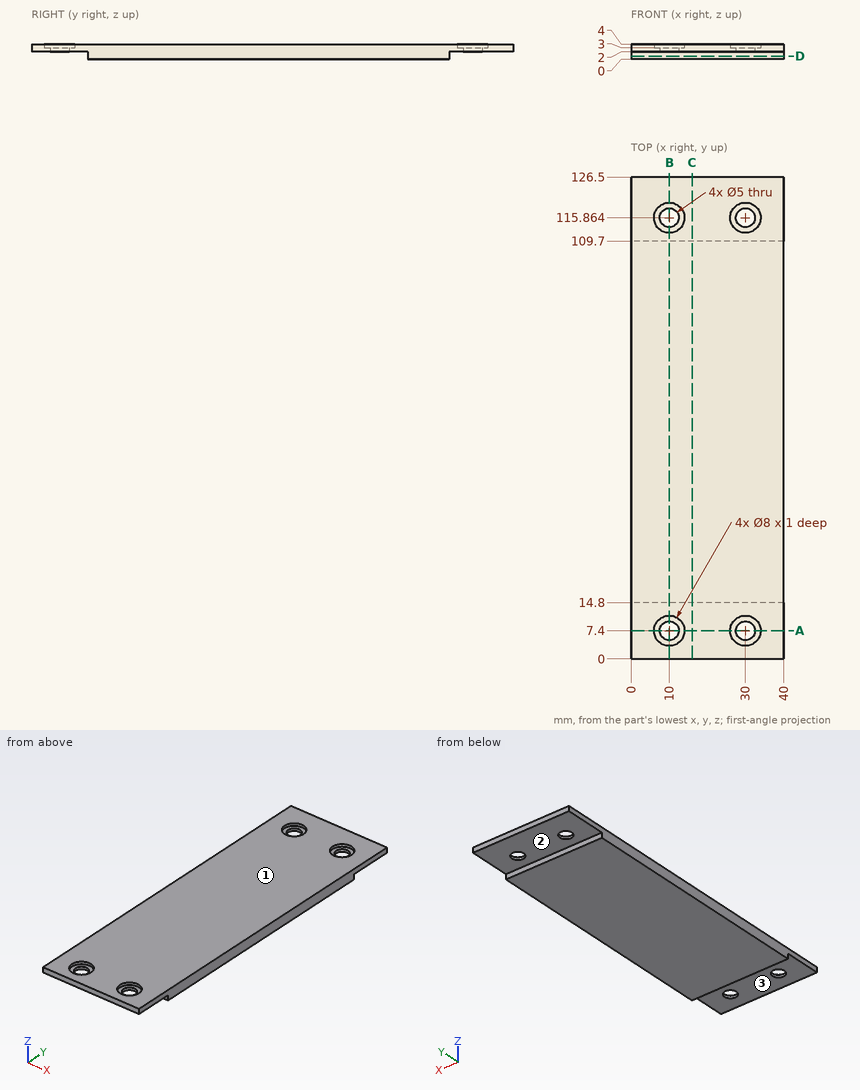
Could you check a few things on this drawing? It's one solid part, dimensions in mm from its lowest x, y, z. A direction names the side the tool comes from. Give positions to 0.01 mm unless a question says otherwise; leave off trailing zeros. Order: outer loops, then holes, each group sorted by start corner. A loop starts at its lowest first (then second) coordinate and runs counter-clockwise, first axis right, second up. Notation, with made-up numbers: (14, 67) - (27, 67) arc R24 cw to (27, 96) - close; hole circle Ø2 at (-1, -10.75). An arc over 180 degrees is marked (long way). One line per question, with ' | ' between items. Start each with the question number.
Item 1: For the marked faces 1, 2 and 3, which set-ups out of +Z, -Z, +X, -X, +Y, -Y let a thin tool reach every point of the face, with its end or its side?
Item 2: I want a section at D-D on z = 0.8. Write out the boundary of the cut face in (x, y), then the cut area to 3 significant figures.
Item 3: I want a section at C-C on x = 16. Write out the boundary of the cut face in (y, z).
Item 4: I want a section at A-A on y = 7.4. Write out the boundary of the cut face in (x, z), then the cut area to 3 significant figures.
Item 5: I want a section at B-B on x = 10. Write out the boundary of the cut face in (y, z).
Item 6: I need wall thicknesses on probe 1 along X at (y, z) = (7.4, 3.5); probe 2 along X at (y, z) = (7.4, 2.45); probe 3 along Y at (x, z) = (13, 3.5). Which ranges of each line are inside material? Lowest first, please. Write a range as [from, to].
Item 7: I'm going to push flat-ended pins straight in: pin 1 Ø6.5 at (x, y) = (10, 115.864) entering from -Z; pin 2 Ø4.5 at (x, y) = (30, 7.4) entering from -Z; pin 3 Ø2.5 at (x, y) = (28.5, 117.5) entering from +Z; pin 4 Ø1.6 at (x, z) = (16, 0.5) entering from +Y. Where does each tip first touch, or does it pass through?
Verdict:
1) face 1: +Z, +X, -X, +Y, -Y | face 2: -Z, +X, -X, +Y | face 3: -Z, +X, -X, -Y
2) outline: (0, 14.8) - (40, 14.8) - (40, 109.7) - (0, 109.7) - close | area: 3,800 mm^2
3) outline: (0, 2) - (14.8, 2) - (14.8, 0) - (109.7, 0) - (109.7, 2) - (126.5, 2) - (126.5, 4) - (0, 4) - close
4) outline: (0, 2) - (7.5, 2) - (7.5, 3) - (6, 3) - (6, 4) - (0, 4) - close; (12.5, 2) - (27.5, 2) - (27.5, 3) - (26, 3) - (26, 4) - (14, 4) - (14, 3) - (12.5, 3) - close; (32.5, 2) - (40, 2) - (40, 4) - (34, 4) - (34, 3) - (32.5, 3) - close | area: 54.0 mm^2
5) outline: (0, 2) - (4.9, 2) - (4.9, 3) - (3.4, 3) - (3.4, 4) - (0, 4) - close; (9.9, 2) - (14.8, 2) - (14.8, 0) - (109.7, 0) - (109.7, 2) - (113.36, 2) - (113.36, 3) - (111.86, 3) - (111.86, 4) - (11.4, 4) - (11.4, 3) - (9.9, 3) - close; (118.36, 2) - (126.5, 2) - (126.5, 4) - (119.86, 4) - (119.86, 3) - (118.36, 3) - close
6) probe 1: [0, 6], [14, 26], [34, 40] | probe 2: [0, 7.5], [12.5, 27.5], [32.5, 40] | probe 3: [0, 4.75], [10.05, 113.22], [118.51, 126.5]
7) pin 1: z = 2 | pin 2: through | pin 3: z = 3 | pin 4: y = 109.7
